Geometry check sheet. Reference: drawing and pictorial views, mm from the part's lowest x, y, z. Round coordinates to 2 decimals unless told otherwise and drop trailing zeros. Write each loop counter-clockwise with the first axis right and the second up, starting at its lowest first coordinate (ties: lowest second). Pieces come first, ordered by that corner, then holes. Notation, with made-up numbers: M 11,47.25 L 69,47.25 A24 cw 69,62.25 Z; hole C -3.75,7 d11. An arc over 180 degrees is marked long. Put each result on its own line as item: value. Start each with the question number.
(1) Material ranges on probe 1 along X at (y, z) = (3, 4.5); probe 2 along X at (y, z) = (3, 3.75); probe 3 along Z at (x, y) = (42.5, 2.6), recorded low to high.
(2) Section check B-B on x = 2.5. Record the cut outline in (y, z).
(3) Section check A-A on y = 3. Record the cut outline in (x, z).
(4) Section check C-C on z = 1. Record the cut outline in (x, y), then the cut area to 3 significant figures.
(5) Gauge pin test, flat end, axial feed: pin 1 (2 mm diameter, centred on x = 42.5, z = 4.5, fed in from +Y). Record the tip position at first contact, or that the pin passes through.
(6) Mould release check, pull along Y, two halves, no side actions. Record for the marked faces 1, 2 and 3: pulls with the +Y half, pulls with the -Y half, needs draft (parallel to the pull), parting line crosses it, or undercut.
(7) Section check D-D on x = 19. Record the cut outline in (y, z), then the cut area to 3 significant figures.
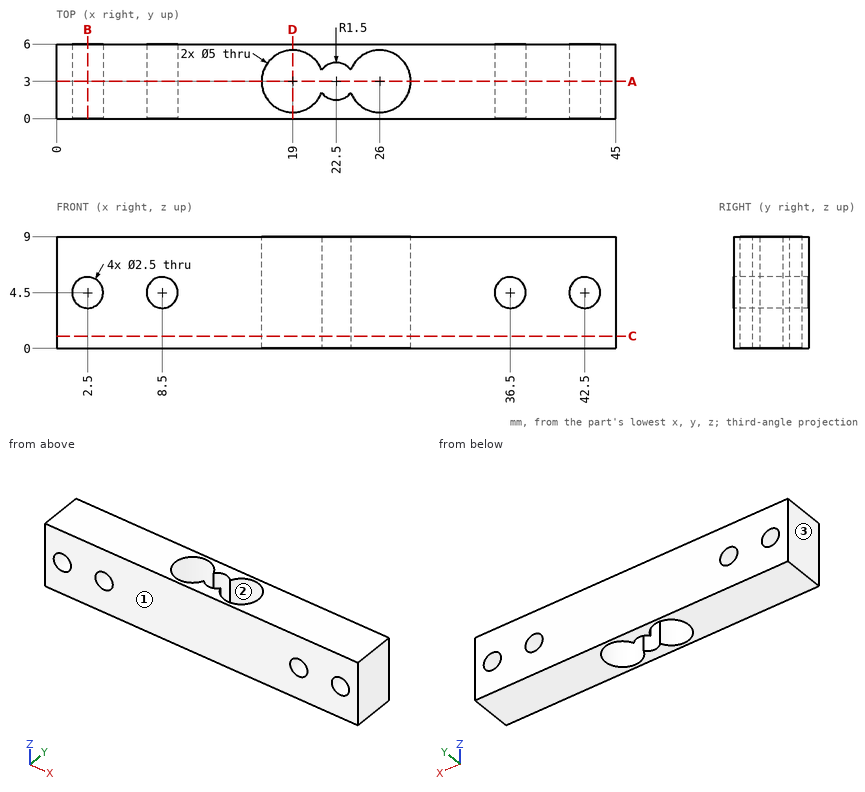
Answers follow:
1. probe 1: x = 0 to 1.25, 3.75 to 7.25, 9.75 to 16.5, 28.5 to 35.25, 37.75 to 41.25, 43.75 to 45
1. probe 2: x = 0 to 1.5, 3.5 to 7.5, 9.5 to 16.5, 28.5 to 35.5, 37.5 to 41.5, 43.5 to 45
1. probe 3: z = 0 to 3.25, 5.75 to 9
2. outline: M 0,0 L 6,0 L 6,3.25 L 0,3.25 Z; M 0,5.75 L 6,5.75 L 6,9 L 0,9 Z
3. outline: M 0,0 L 16.5,0 L 16.5,9 L 0,9 Z; M 28.5,0 L 45,0 L 45,9 L 28.5,9 Z; hole C 2.5,4.5 d2.5; hole C 8.5,4.5 d2.5; hole C 36.5,4.5 d2.5; hole C 42.5,4.5 d2.5
4. outline: M 0,0 L 45,0 L 45,6 L 0,6 Z; hole M 21.32,2.07 A1.5 ccw 23.68,2.07 A2.5 ccw long 23.68,3.93 A1.5 ccw 21.32,3.93 A2.5 ccw long Z
4. area: 225 mm^2
5. pin 1: passes through
6. face 1: pulls with the -Y half
6. face 2: undercut
6. face 3: needs draft
7. outline: M 0,0 L 0.5,0 L 0.5,9 L 0,9 Z; M 5.5,0 L 6,0 L 6,9 L 5.5,9 Z
7. area: 9.00 mm^2
